Here's how the part is built. I have some questions about the finished solid (model axes, mm). Face numbers are marked on the shaded views. Round coordinates to 2 decimals unless told otherwise and drop trailing zeros. Loops run counter-clockwise (first coordinate to the right, second up) from the corner with the lowest first, then second, coordinate; pieces in that order, holes last. Notation, with made-up numbers: M 1.5,13 L 23.5,13 A19 ccw 23.5,29 Z; hole C 66.5,43 d2. An arc over 180 degrees is marked long. Use a Markdown table: item, result.
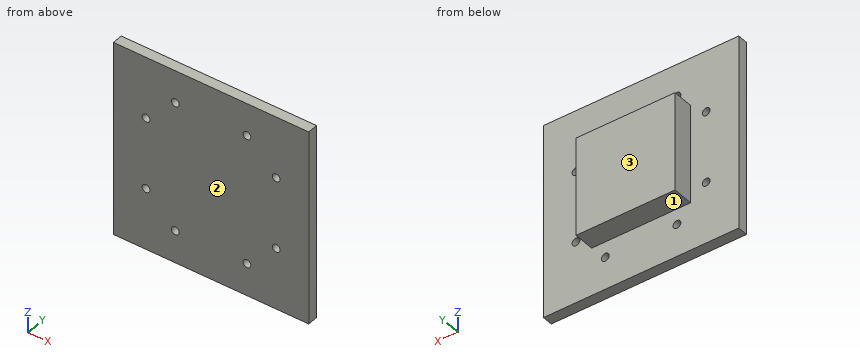
from build123d import *

# Parameters (mm, degrees)
SKETCH1_W           = 30
SKETCH1_H           = 30
BOSS_EXTRUDE1_DEPTH = 1.6
SKETCH2_R           = 0.6
CUT_EXTRUDE1_DEPTH  = 1.6
CIRPATTERN1_COUNT   = 2
CIRPATTERN1_ANGLE   = 90
SKETCH4_W           = 15.2
SKETCH4_H           = 15.2
BOSS_EXTRUDE2_DEPTH = 3.2


with BuildPart() as part:
    # Sketch1 → Boss-Extrude1 (new body)
    with BuildSketch(Plane(origin=(0, 0, 0), x_dir=(1, 0, 0), z_dir=(0, 1, 0))):
        with Locations((15, 15)):
            Rectangle(SKETCH1_W, SKETCH1_H)
    extrude(amount=BOSS_EXTRUDE1_DEPTH)

    # Sketch2 → Cut-Extrude1 (cut)
    with BuildSketch(Plane(origin=(0, 1.6, 0), x_dir=(1, 0, 0), z_dir=(0, 1, 0))):
        with Locations((20.5, 5)):
            Circle(SKETCH2_R)
        with Locations((9.5, 5)):
            Circle(SKETCH2_R)
        with Locations((20.5, 25)):
            Circle(SKETCH2_R)
        with Locations((9.5, 25)):
            Circle(SKETCH2_R)
    cut_extrude1 = extrude(amount=-CUT_EXTRUDE1_DEPTH, mode=Mode.SUBTRACT)

    # CirPattern1: Cut-Extrude1 ×2 about axis
    cirpattern1_axis = Axis((15, 0, -15), (0, 1, 0))
    for i in range(1, CIRPATTERN1_COUNT):
        add(cut_extrude1.rotate(cirpattern1_axis, i * CIRPATTERN1_ANGLE / (CIRPATTERN1_COUNT - 1)), mode=Mode.SUBTRACT)

    # Sketch4 → Boss-Extrude2 (add)
    with BuildSketch(Plane(origin=(0, 1.6, 0), x_dir=(1, 0, 0), z_dir=(0, 1, 0))):
        with Locations((15, 15)):
            Rectangle(SKETCH4_W, SKETCH4_H)
    extrude(amount=BOSS_EXTRUDE2_DEPTH)


solid = part.part
1. Imagine slicing it at A-A, the plane x = 25. Write out the boundary of the cut face in (y, z).
Answer sheet:
| item | result |
|---|---|
| outline | M 0,-30 L 1.6,-30 L 1.6,-21.1 L 0,-21.1 Z; M 0,-19.9 L 1.6,-19.9 L 1.6,-10.1 L 0,-10.1 Z; M 0,-8.9 L 1.6,-8.9 L 1.6,0 L 0,0 Z |
2. Imagine slicing it at C-C, the plane z = -22.25. Write out the boundary of the cut face in (x, y), then the cut area to 3 significant figures.
Answer sheet:
| item | result |
|---|---|
| outline | M 0,0 L 30,0 L 30,1.6 L 22.6,1.6 L 22.6,4.8 L 7.4,4.8 L 7.4,1.6 L 0,1.6 Z |
| area | 96.6 mm2 |
3. Imagine slicing it at D-D, the plane x = 9.5. Write out the boundary of the cut face in (y, z), then the cut area to 3 significant figures.
Answer sheet:
| item | result |
|---|---|
| outline | M 0,-30 L 1.6,-30 L 1.6,-25.6 L 0,-25.6 Z; M 0,-24.4 L 1.6,-24.4 L 1.6,-22.6 L 4.8,-22.6 L 4.8,-7.4 L 1.6,-7.4 L 1.6,-5.6 L 0,-5.6 Z; M 0,-4.4 L 1.6,-4.4 L 1.6,0 L 0,0 Z |
| area | 92.8 mm2 |
4. I need wall thicknesses on probe 1 along X at (y, z) = (0.7, -5); probe 2 along Z at (x, y) = (9.5, 0.7); probe 3 along X at (y, z) = (0.9, -20.5). Which ranges of each line are inside material? Lowest first, please. Write a range as from..to.
Answer sheet:
| item | result |
|---|---|
| probe 1 | 0..8.9, 10.1..19.9, 21.1..30 |
| probe 2 | -30..-25.6, -24.4..-5.6, -4.4..0 |
| probe 3 | 0..4.4, 5.6..24.4, 25.6..30 |
5. We'd pull the mould along Y, two halves only. Please class the marked faces 1, 2 and 3: +Y half, -Y half, draft (parallel to the pull), parting line (faces both ways), or undercut.
Answer sheet:
| item | result |
|---|---|
| face 1 | draft |
| face 2 | -Y half |
| face 3 | +Y half |
6. Imagine slicing it at B-B, the plane z = -9.5. Write out the boundary of the cut face in (x, y).
Answer sheet:
| item | result |
|---|---|
| outline | M 0,0 L 4.4,0 L 4.4,1.6 L 0,1.6 Z; M 5.6,0 L 24.4,0 L 24.4,1.6 L 22.6,1.6 L 22.6,4.8 L 7.4,4.8 L 7.4,1.6 L 5.6,1.6 Z; M 25.6,0 L 30,0 L 30,1.6 L 25.6,1.6 Z |
7. For pin 1 Ø1.5 at (x, y) = (24, 4) entering from -Z; pin 2 Ø1.4 at (x, z) = (5, -20.5) entering from +Y; pin 3 Ø1.6 at (y, z) = (3.5, -17) entering from -X; pin 4 Ø2.5 at (x, y) = (15.5, 4) entering from +Z, each with a flat end and sliding along its axis, tell me the tip position at first contact or that it passes through.
Answer sheet:
| item | result |
|---|---|
| pin 1 | through |
| pin 2 | y = 1.6 |
| pin 3 | x = 7.4 |
| pin 4 | z = -7.4 |
